from build123d import *

# Parameters (mm, degrees)
F0_W     = 28
F0_H     = 45
F1_DEPTH = 19
F2_D     = 5
F3_W     = 26
F3_H     = 17
F4_DEPTH = 45.001
F6_D     = 3.3
F7_W     = 17.5
F7_H     = 6
F8_DEPTH = 28.001


with BuildPart() as f1:
    # F0 (on Top) → F1 (new body)
    with BuildSketch(Plane.XY):
        with Locations((-1.5, 0)):
            Rectangle(F0_W, F0_H)
    extrude(amount=F1_DEPTH)

    # F2 (through all)
    with Locations(Plane(origin=(0, 0, 0), x_dir=(1, 0, 0), z_dir=(0, 0, -1))):
        with Locations((8, 2), (-8, 2), (-8, 18), (8, 18)):
            Hole(F2_D / 2)

    # F3 (on face) → F4 (cut, through all)
    with BuildSketch(Plane.XZ.offset(22.5)):
        with Locations((-0.5, 8.5)):
            Rectangle(F3_W, F3_H)
    extrude(amount=-F4_DEPTH, mode=Mode.SUBTRACT)

    # F6 (through all)
    with Locations(Plane(origin=(-15.5, 0, 0), x_dir=(0, -1, 0), z_dir=(-1, 0, 0))):
        with Locations((-18.5, 7.5), (18.5, 7.5)):
            Hole(F6_D / 2)

    # F7 (on face) → F8 (cut, through all)
    with BuildSketch(Plane(origin=(-15.5, 0, 0), x_dir=(0, -1, 0), z_dir=(-1, 0, 0))):
        with Locations((-13.75, 16)):
            Rectangle(F7_W, F7_H)
    extrude(amount=-F8_DEPTH, mode=Mode.SUBTRACT)


solid = f1.part
The model under review builds one solid part; all positions refer to its coordinate system, in mm. A direction names the side the tool comes from. Round coordinates to 2 decimals unless told otherwise and drop trailing zeros. Loops run counter-clockwise (first coordinate to the right, second up) from the corner with the lowest first, then second, coordinate; pieces in that order, holes last. Notation, with made-up numbers: M 70,40 L 117,40 A10 cw 117,53 Z; hole C -4.75,9.25 d5. An arc over 180 degrees is marked long. Answer as CSV lines item,"result". Start each with the question number.
Item 1: Consider section B-B (x = 10). Write out the cut boundary in (y, z), then the cut area to 3 significant figures.
Item 2: For faces 1 (the face through (-15, 14, 13)), 2 (the face through (-9.34, -20.11, 18.01)), 3 (the face through (-13.5, 0, 8)), list the 3-axis set-ups (+Z, -Z, +X, -X, +Y, -Y) from which the entire face can be reached by the end or side of a thin tool; tool diameter is ignored.
Item 3: Insertion check: P1, Ø1, axis at x = -14, y = 14.5, coming from the +Z side; P2, Ø4.5, axis at x = -8, y = -2, coming from the +Z side; P3, Ø5, axis at x = 1.5, z = 16.5, coming from the +Y side; P4, Ø13, axis at x = -5, y = -4.5, coming from the -Z side. Each pin has a flat end and moves straight along its axis. Give the tip position at first contact, or say it passes through.
Item 4: Wall thickness on line 1 (Y direction, x = 8, z = 18.35); line 2 (X direction, y = -18, z = 18.4); line 3 (X direction, y = -6.5, z = 12.5): over which ranges is each line inside the solid? List them lowest first. Write a range as [from, to].
Item 5: Mouldability with a two-part tool opening along Y and no side actions: class faces 4 (the face through (-4.8, 5, 17.3)), 5 (the face through (-10.385, -2.751, 18.014)), 6 (the face through (-6.8, -22.5, 17.2)) as released by +Y, released by -Y, zero draft, split by the parting line, or undercut.
Item 6: Consider section A-A (y = -2). Write out the cut boundary in (x, z), then the cut area to 3 significant figures.
Item 7: Consider section D-D (x = -8). Write out the cut boundary in (y, z).
Item 8: Consider section C-C (y = -18.5). Write out the cut boundary in (x, z).
Answer:
1,outline,"M -22.5,17 L -19.5,17 L -19.5,19 L -22.5,19 Z; M -16.5,17 L -3.5,17 L -3.5,19 L -16.5,19 Z; M -0.5,17 L 5,17 L 5,19 L -0.5,19 Z"
1,area,"43.0 mm^2"
2,face 1,"+Z, +X, -X, +Y"
2,face 2,"+Z, -Z"
2,face 3,"-Z, +X, +Y, -Y"
3,P1,"stops at z = 13"
3,P2,"passes through"
3,P3,"stops at y = 5"
3,P4,"stops at z = 17"
4,line 1,"y = [-22.5, -20.5], [-15.5, -4.5], [0.5, 5]"
4,line 2,"x = [-15.5, -10.5], [-5.5, 5.5], [10.5, 12.5]"
4,line 3,"x = [-15.5, -13.5]"
5,face 4,"released by +Y"
5,face 5,"undercut"
5,face 6,"released by -Y"
6,outline,"M -15.5,0 L -13.5,0 L -13.5,17 L -10.5,17 L -10.5,19 L -15.5,19 Z; M -5.5,17 L 5.5,17 L 5.5,19 L -5.5,19 Z; M 10.5,17 L 12.5,17 L 12.5,19 L 10.5,19 Z"
6,area,"70.0 mm^2"
7,outline,"M -22.5,17 L -20.5,17 L -20.5,19 L -22.5,19 Z; M -15.5,17 L -4.5,17 L -4.5,19 L -15.5,19 Z; M 0.5,17 L 5,17 L 5,19 L 0.5,19 Z"
8,outline,"M -15.5,0 L -13.5,0 L -13.5,5.85 L -15.5,5.85 Z; M -15.5,9.15 L -13.5,9.15 L -13.5,17 L -10.45,17 L -10.45,19 L -15.5,19 Z; M -5.55,17 L 5.55,17 L 5.55,19 L -5.55,19 Z; M 10.45,17 L 12.5,17 L 12.5,19 L 10.45,19 Z"
